from build123d import *

# Parameters (mm, degrees)
F0_W     = 27
F0_H     = 117
F0_W_2   = 25
F0_H_2   = 99
F1_DEPTH = 88
F2_DEPTH = 1
F3_W     = 54
F3_H     = 2.5
F4_DEPTH = 82
F5_W     = 35
F5_H     = 7
F6_DEPTH = 54


with BuildPart() as f1:
    # F0 (on Top) → F1 (new body)
    with BuildSketch(Plane.XY):
        with Locations((-13.5, 0)):
            Rectangle(F0_W, F0_H)
        with Locations((-13.5, 1)):
            Rectangle(F0_W_2, F0_H_2, mode=Mode.SUBTRACT)
        with Locations((13.5, 0)):
            Rectangle(F0_W, F0_H)
        with Locations((13.5, 1)):
            Rectangle(F0_W_2, F0_H_2, mode=Mode.SUBTRACT)
        with Locations((-13.5, 1)):
            Rectangle(F0_W_2, F0_H_2)
        with Locations((13.5, 1)):
            Rectangle(F0_W_2, F0_H_2)
    extrude(amount=-F1_DEPTH)

    # F0 (on Top) → F2 (cut)
    with BuildSketch(Plane.XY):
        with Locations((-13.5, 1)):
            Rectangle(F0_W_2, F0_H_2)
        with Locations((13.5, 1)):
            Rectangle(F0_W_2, F0_H_2)
    extrude(amount=-F2_DEPTH, mode=Mode.SUBTRACT)

    # F3 (on face) → F4 (cut)
    with BuildSketch(Plane(origin=(0, 0, -88), x_dir=(1, 0, 0), z_dir=(0, 0, -1))):
        with Locations((0, 57.25)):
            Rectangle(F3_W, F3_H)
        with Locations((0, -57.25)):
            Rectangle(F3_W, F3_H)
    extrude(amount=-F4_DEPTH, mode=Mode.SUBTRACT)

    # F5 (on face) → F6 (cut, through all)
    with BuildSketch(Plane.YZ.offset(27)):
        with Locations((-3.5, -84.5)):
            Rectangle(F5_W, F5_H)
    extrude(amount=-F6_DEPTH, mode=Mode.SUBTRACT)


solid = f1.part
Could you check a few things on this model? Use its own coordinates, in mm. A direction names the side the tool comes from. Coordinates: 2 decimals unless noted, no trailing zeros. Loops run counter-clockwise (first coordinate to the right, second up) from the corner with the lowest first, then second, coordinate; pieces in that order, holes last.
1. For P1, Ø7.5, axis at x = 12, y = 6.5, coming from the +Z side; P2, Ø1.2, axis at x = -13.5, y = -57, coming from the -Z side; P3, Ø1, axis at x = 5.5, y = 9, coming from the -Z side, each with a flat end and sliding along its axis, tell me the tip position at first contact or that it passes through.
2. We'd pull the mould along X, two halves only. Please class faces 4 (the face through (-14, 2, -1)), 5 (the face through (0, -58.5, -3)), 6 (the face through (-27, -1, -43)): released by +X, released by -X, zero draft, split by the parting line, or undercut.
3. Imagine slicing it at B-B (y = -3). Please give me the cut outline in (x, z).
4. Imagine slicing it at A-A (x = 23.5). Please give me the cut outline in (y, z).
5. I need wall thicknesses on L1, parallel to Z at x = 22.5, y = -30; L2, parallel to Y at x = -25, z = -52; L3, parallel to Z at x = -18, y = 2. Which ranges of each line are inside material? Lowest first, please.
6. For faces 1 (the face through (13, 2, -1)), 2 (the face through (0, 57, -6)), 3 (the face through (0, 14, -85)), which set-ups out of +Z, -Z, +X, -X, +Y, -Y let a thin tool reach every point of the face, with its end or its side?
7. Imagine slicing it at C-C (z = -67.5). Please give me the cut outline in (x, y).
Computed values:
1. P1: stops at z = -1
1. P2: stops at z = -6
1. P3: stops at z = -81
2. face 4: undercut
2. face 5: zero draft
2. face 6: released by -X
3. outline: (-27, -81) - (27, -81) - (27, 0) - (26, 0) - (26, -1) - (1, -1) - (1, 0) - (-1, 0) - (-1, -1) - (-26, -1) - (-26, 0) - (-27, 0) - close
4. outline: (-58.5, -6) - (-56, -6) - (-56, -88) - (-21, -88) - (-21, -81) - (14, -81) - (14, -88) - (56, -88) - (56, -6) - (58.5, -6) - (58.5, 0) - (50.5, 0) - (50.5, -1) - (-48.5, -1) - (-48.5, 0) - (-58.5, 0) - close
5. L1: z = -88 to -1
5. L2: y = -56 to 56
5. L3: z = -81 to -1
6. face 1: +Z
6. face 2: -Z, +X, -X, +Y
6. face 3: -Z, +X, -X
7. outline: (-27, -56) - (27, -56) - (27, 56) - (-27, 56) - close
